Autodesk Inventor part; units mm, degrees
ref_plane "YZ Plane" through (0, 0, 0) normal (1, 0, 0) x (0, 1, 0)
ref_plane "XZ Plane" through (0, 0, 0) normal (0, 1, 0) x (-1, 0, 0)
ref_plane "XY Plane" through (0, 0, 0) normal (0, 0, 1) x (1, 0, 0)
sketch "Sketch1" plane through (0, 0, 0) normal (0, 0, 1) x (1, 0, 0)
  line L0 (18.8411, 66.8659) -> (163.8411, 66.8659)
  line L1 (163.8411, 66.8659) -> (163.8411, 11.8659)
  line L2 (163.8411, 11.8659) -> (18.8411, 11.8659)
  line L3 (18.8411, 11.8659) -> (18.8411, 66.8659)
  point P0 (0, 0)
  dimension "d0" = 55
  dimension "d1" = 145
extrude "Extrusion1" add sketch "Sketch1" along normal blind 35
sketch "Sketch2" plane through (0, 0, 35) normal (0, 0, 1) x (1, 0, 0)
  line L0 (23.8411, 61.8659) -> (158.8411, 61.8659)
  line L1 (158.8411, 61.8659) -> (158.8411, 16.8659)
  line L2 (158.8411, 16.8659) -> (23.8411, 16.8659)
  line L3 (23.8411, 16.8659) -> (23.8411, 61.8659)
  line L4 (18.8411, 66.8659) -> (18.8411, 11.8659)
  line L5 (163.8411, 66.8659) -> (18.8411, 66.8659)
  line L6 (163.8411, 11.8659) -> (163.8411, 66.8659)
  line L7 (18.8411, 11.8659) -> (163.8411, 11.8659)
  point P0 (0, 0)
  dimension "d4" = 5
  dimension "d5" = 5
  dimension "d6" = 5
  dimension "d7" = 5
extrude "Extrusion2" cut sketch "Sketch2" against normal blind 30 contours L0 L1 L2 L3
sketch "Sketch3" plane through (0, 0, 0) normal (0, 0, -1) x (-1, 0, 0)
  circle A0 centre (-29.8411, 22.8659) radius 1.5
  circle A1 centre (-29.8411, 55.8659) radius 1.5
  line L0 (-18.8411, 66.8659) -> (-18.8411, 11.8659)
  line L1 (-18.8411, 11.8659) -> (-163.8411, 11.8659)
  line L2 (-163.8411, 66.8659) -> (-18.8411, 66.8659)
  circle A2 centre (-127.8411, 55.8659) radius 1.5
  circle A3 centre (-127.8411, 22.8659) radius 1.5
  line L3 (-163.8411, 11.8659) -> (-163.8411, 66.8659)
  circle A4 centre (-115.8411, 55.8659) radius 1.5
  circle A5 centre (-115.8411, 22.8659) radius 1.5
  point P0 (0, 0)
  dimension "d10" = 3
  dimension "d11" = 11
  dimension "d12" = 11
  dimension "d13" = 11
  dimension "d14" = 11
  dimension "d15" = 3
  dimension "d19" = 3
  dimension "d20" = 3
  dimension "d24" = 36
  dimension "d26" = 12
  dimension "d27" = 36
  dimension "d28" = 12
  dimension "d29" = 3
  dimension "d30" = 3
  dimension "d31" = 11
  dimension "d32" = 11
  dimension "d33" = 11
  dimension "d34" = 11
extrude "Extrusion3" cut sketch "Sketch3" against normal blind 30 contours A0 | A1 | A2 | A3 | A4 | A5
sketch "Sketch4" plane through (18.8411, 11.8659, 0) normal (-1, 0, 0) x (0, 0, 1)
  line L0 (35, 0) -> (35, 55)
  line L1 (35, 48) -> (15, 48)
  line L2 (15, 48) -> (15, 18)
  line L3 (15, 18) -> (35, 18)
  line L4 (35, 18) -> (35, 48)
  line L5 (0, 55) -> (35, 55)
  line L6 (15, 20) -> (15, 40)
  line L7 (15, 45) -> (5, 45)
  line L8 (5, 45) -> (5, 20)
  line L9 (5, 20) -> (15, 20)
  line L10 (15, 20) -> (15, 45)
  line L11 (0, 55) -> (0, 0)
  point P0 (0, -11.8659)
  point P1 (35, 18)
  point P2 (15, 20)
  point P3 (15, 20)
  dimension "d37" = 7
  dimension "d38" = 30
  dimension "d44" = 10
  dimension "d45" = 25
  dimension "d46" = 5
  dimension "d47" = 15
extrude "Extrusion4" cut sketch "Sketch4" against normal blind 30
sketch "Sketch5" plane through (163.8411, 11.8659, 0) normal (1, 0, 0) x (0, 0, -1)
  circle A0 centre (-13, 17) radius 2
  circle A1 centre (-13, 42) radius 2
  line L0 (0, 0) -> (0, 55)
  line L1 (0, 0) -> (-35, 0)
  dimension "d48" = 4
  dimension "d49" = 4
  dimension "d50" = 25
  dimension "d51" = 13
  dimension "d52" = 13
  dimension "d53" = 17
extrude "Extrusion5" cut sketch "Sketch5" against normal blind 30
properties part number "arduino mould_thicker"
For this review, take the finished solid that the model builds, in its own axes (mm). A direction names the side the tool comes from. Round coordinates to 2 decimals unless told otherwise and drop trailing zeros. Write each loop counter-clockwise with the first axis right and the second up, starting at its lowest first coordinate (ties: lowest second). Pieces come first, ordered by that corner, then holes.
1) Take a section at D-D on z = 26. Give the boundary of the cut face in (x, y), then the cut area to 3 significant figures.
Answer below:
outline: (18.84, 11.87) - (163.84, 11.87) - (163.84, 66.87) - (18.84, 66.87) - (18.84, 59.87) - (23.84, 59.87) - (23.84, 61.87) - (158.84, 61.87) - (158.84, 16.87) - (23.84, 16.87) - (23.84, 29.87) - (18.84, 29.87) - close
area: 1,750 mm2
2) Take a section at C-C on x = 52.5. Give the boundary of the cut face in (y, z), then the cut area to 3 significant figures.
Answer below:
outline: (11.87, 0) - (66.87, 0) - (66.87, 35) - (61.87, 35) - (61.87, 5) - (16.87, 5) - (16.87, 35) - (11.87, 35) - close
area: 575 mm2
3) Take a section at A-A on z = 13. Give the boundary of the cut face in (x, y).
Answer below:
outline: (18.84, 11.87) - (163.84, 11.87) - (163.84, 26.87) - (158.84, 26.87) - (158.84, 16.87) - (23.84, 16.87) - (23.84, 31.87) - (18.84, 31.87) - close; (18.84, 56.87) - (23.84, 56.87) - (23.84, 61.87) - (158.84, 61.87) - (158.84, 55.87) - (163.84, 55.87) - (163.84, 66.87) - (18.84, 66.87) - close; (158.84, 30.87) - (163.84, 30.87) - (163.84, 51.87) - (158.84, 51.87) - close
4) Mouldability with a two-part tool opening along X and no side actions: class faces 1 (the face through (18.841, 27, 13)), 2 (the face through (158.841, 40, 20)), 3 (the face through (21, 59.866, 25)) as +X half, -X half, draft (parallel to the pull), parting line (faces both ways), or undercut.
Answer below:
face 1: -X half
face 2: undercut
face 3: draft
5) Take a section at B-B on y = 18.5. Give the boundary of the cut face in (x, z), then the cut area to 4 significant figures.
Answer below:
outline: (18.84, 0) - (163.84, 0) - (163.84, 35) - (158.84, 35) - (158.84, 5) - (23.84, 5) - (23.84, 35) - (18.84, 35) - close
area: 1,025 mm2
6) Machinability: for faces 4 (the face through (161.376, 26.913, 13.434)), 5 (the face through (90, 61.866, 20)), 6 (the face through (21, 31.866, 10)), 7 (the face through (31.34, 55.93, 2.46)), 8 (the face through (161.38, 55.85, 13.26)), which of the approach directions +Z, -Z, +X, -X, +Y, -Y give a long, thin tool a straight path to every point of the face, cutting with its end or side? Answer none if there is none.
Answer below:
face 4: +X
face 5: +Z
face 6: +Z, -X
face 7: +Z, -Z
face 8: +X, -X
7) For line 1 along Y through (x, z) = (160, 13); line 2 along X through (y, z) = (27, 29.5); line 3 along Y through (x, z) = (142.5, 22), list the stretches that pass through material, from the lowest coordinate up.
Answer below:
line 1: y = 11.87 to 26.87, 30.87 to 51.87, 55.87 to 66.87
line 2: x = 18.84 to 23.84, 158.84 to 163.84
line 3: y = 11.87 to 16.87, 61.87 to 66.87
8) Insertion check: pin 1 Ø5 at (x, y) = (115.84, 22.87) entering from +Z; pin 2 Ø2 at (x, y) = (22.5, 31) entering from +Z. Each pin has a flat end and moves straight along its axis. Give the tip position at first contact, or say it passes through.
Answer below:
pin 1: stops at z = 5
pin 2: stops at z = 15
